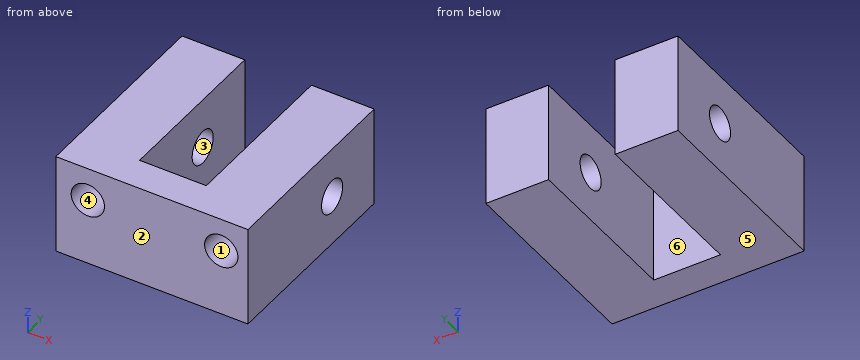
```python
from build123d import *

# Parameters (mm, degrees)
BOSS_EXTRUDE1_DEPTH = 9.525
HOLE1_D             = 6.35
HOLE2_D             = 6.35
HOLE2_DEPTH         = 12.7


with BuildPart() as part:
    # Sketch1 → Boss-Extrude1 (new, symmetric)
    with BuildSketch(Plane.XY):
        Polygon((-18.288, 0), (-18.288, 38.1), (-6.35, 38.1), (-6.35, 6.35), (6.35, 6.35), (6.35, 38.1), (18.288, 38.1), (18.288, 0), align=None)
    extrude(amount=BOSS_EXTRUDE1_DEPTH, both=True)

    # Hole1 (through all)
    with Locations(Plane(origin=(18.288, 0, 0), x_dir=(0, 0, -1), z_dir=(1, 0, 0))):
        with Locations((0, 25.4)):
            Hole(HOLE1_D / 2)

    # Hole2
    with Locations(Plane(origin=(0, 0, 0), x_dir=(-1, 0, 0), z_dir=(0, -1, 0))):
        with Locations((-13.208, -3.175), (12.192, -3.175)):
            Hole(HOLE2_D / 2, depth=HOLE2_DEPTH)


solid = part.part
```
Could you check a few things on this model? Use its own coordinates, in mm. Face numbers are marked on the shaded views. A direction names the side the tool comes from. Round coordinates to 2 decimals unless told otherwise and drop trailing zeros. Loops run counter-clockwise (first coordinate to the right, second up) from the corner with the lowest first, then second, coordinate; pieces in that order, holes last.
Q1. I want a section at A-A (y = 21). Write out the boundary of the cut face in (x, z) (3 decimals).
Q2. I want a section at D-D (z = 0.5). Write out the boundary of the cut face in (x, y).
Q3. On a 3-axis mill with a long thin cutter (end or side, diameter ignored), from which of +Z, -Z, +X, -X, +Y, -Y can I reach the whole of each face in a straight line? I mean the marked faces 4, 5 and 6. Say none if no direction works.
Q4. I want a section at B-B (y = 25.4). Write out the boundary of the cut face in (x, z) (3 decimals).
Q5. I want a section at C-C (x = -7). Write out the boundary of the cut face in (y, z) (3 decimals), and give its area (3 significant figures).
Q6. For P1, Ø3, axis at x = -12, z = 3, coming from the -Y side, with a flat end and sliding along its axis, tell me the tip position at first contact or that it passes through.
Q7. Thinking about a two-plate mould opening in Y: for the marked faces 1, 2 and 3, which applies, pulls with the +Y half, pulls with the -Y half, needs draft (parallel to the pull), parting line crosses it, or undercut?
Q8. Please list where these lines run through material, in increasing order: L1, parallel to X at y = 33.5, z = -4; L2, parallel to X at y = 11.5, z = 5.25.
Answer below:
1. outline: (-18.288, -9.525) - (-6.35, -9.525) - (-6.35, 9.525) - (-18.288, 9.525) - close; (6.35, -9.525) - (18.288, -9.525) - (18.288, 9.525) - (6.35, 9.525) - close
2. outline: (-18.29, 0) - (-13.9, 0) - (-13.9, 12.7) - (-10.48, 12.7) - (-10.48, 0) - (11.5, 0) - (11.5, 12.7) - (14.92, 12.7) - (14.92, 0) - (18.29, 0) - (18.29, 22.26) - (6.35, 22.26) - (6.35, 6.35) - (-6.35, 6.35) - (-6.35, 22.26) - (-18.29, 22.26) - close; (-18.29, 28.54) - (-6.35, 28.54) - (-6.35, 38.1) - (-18.29, 38.1) - close; (6.35, 28.54) - (18.29, 28.54) - (18.29, 38.1) - (6.35, 38.1) - close
3. face 4: -Y
3. face 5: -Z, +X, -X, +Y, -Y
3. face 6: +Z, -Z, +Y
4. outline: (-18.288, -9.525) - (-6.35, -9.525) - (-6.35, -3.175) - (-18.288, -3.175) - close; (-18.288, 3.175) - (-6.35, 3.175) - (-6.35, 9.525) - (-18.288, 9.525) - close; (6.35, -9.525) - (18.288, -9.525) - (18.288, -3.175) - (6.35, -3.175) - close; (6.35, 3.175) - (18.288, 3.175) - (18.288, 9.525) - (6.35, 9.525) - close
5. outline: (0, -9.525) - (38.1, -9.525) - (38.1, 9.525) - (0, 9.525) - close; hole circle Ø6.35 at (25.4, 0)
5. area: 694 mm2
6. P1: stops at y = 12.7
7. face 1: needs draft
7. face 2: pulls with the -Y half
7. face 3: undercut
8. L1: x = -18.29 to -6.35, 6.35 to 18.29
8. L2: x = -18.29 to -14.6, -9.79 to -6.35, 6.35 to 10.8, 15.61 to 18.29
